Build history of the part. All positions in model axes, mm. A direction names the side the tool comes from. Round coordinates to 2 decimals unless told otherwise and drop trailing zeros. Write each loop counter-clockwise with the first axis right and the second up, starting at its lowest first coordinate (ties: lowest second). Pieces come first, ordered by that corner, then holes. Notation, with made-up numbers: (-28.5, 45) - (15.5, 45) arc R10 ccw to (15.5, 49) - close; hole circle Ø10 at (43.5, 37). An arc over 180 degrees is marked (long way). Write each question's results on one line, items separated by ' | '.
from build123d import *

# Parameters (mm, degrees)
SKETCH_1_W          = 70
SKETCH_1_H          = 70
EXTRUDE_1_DEPTH     = 50
SKETCH_2_W          = 55
SKETCH_2_H          = 55
CUT_EXTRUDE_1_DEPTH = 50


with BuildPart() as part:
    # 草图1 → 凸台-拉伸1 (new body)
    with BuildSketch(Plane(origin=(0, 0, 0), x_dir=(1, 0, 0), z_dir=(0, 1, 0))):
        Rectangle(SKETCH_1_W, SKETCH_1_H)
    extrude(amount=-EXTRUDE_1_DEPTH)

    # 草图2 → 切除-拉伸1 (cut)
    with BuildSketch(Plane(origin=(0, 0, 0), x_dir=(1, 0, 0), z_dir=(0, 1, 0))):
        Rectangle(SKETCH_2_W, SKETCH_2_H)
    extrude(amount=-CUT_EXTRUDE_1_DEPTH, mode=Mode.SUBTRACT)


solid = part.part
(1) Slice it at A-A, the plane z = -16. Write the cut outline in (x, y).
Worked answers:
outline: (-35, -50) - (-27.5, -50) - (-27.5, 0) - (-35, 0) - close; (27.5, -50) - (35, -50) - (35, 0) - (27.5, 0) - close
(2) Slice it at C-C, the plane y = -5.5. Write the cut outline in (x, z), and give its area (4 significant figures).
Worked answers:
outline: (-35, -35) - (35, -35) - (35, 35) - (-35, 35) - close; hole (-27.5, -27.5) - (27.5, -27.5) - (27.5, 27.5) - (-27.5, 27.5) - close | area: 1,875 mm2
(3) Tool access for faces 5 (the flat face through (27.5, -25, 0)), 6 (the flat face through (0, -25, 35)): list every direction of +Z, -Z, +X, -X, +Y, -Y with a clear straight run to the whole face (end or side of a thin tool).
Worked answers:
face 5: +Y, -Y | face 6: +Z, +X, -X, +Y, -Y
(4) Drill centre line: probe 1 along Z at (x, y) = (2.5, -41.5). Where is it in solid material? Low to high. Write a range as [from, to].
Worked answers:
probe 1: z = [-35, -27.5], [27.5, 35]
(5) Slice it at B-B, the plane x = 19.5. Write the cut outline in (y, z).
Worked answers:
outline: (-50, -35) - (0, -35) - (0, -27.5) - (-50, -27.5) - close; (-50, 27.5) - (0, 27.5) - (0, 35) - (-50, 35) - close
(6) Two-plate mould, pull along X, no slides. Class faces 1 (the flat face through (-32, 0, 0)), 2 (the flat face through (35, -25, 0)), 3 (the flat face through (0, -25, 27.5)), 4 (the flat face through (0, -25, -27.5)): released by +X, released by -X, zero draft, split by the parting line, or undercut.
Worked answers:
face 1: zero draft | face 2: released by +X | face 3: undercut | face 4: undercut
